Model file for the job. Use its own axes, mm. A direction names the side the tool comes from. Round coordinates to 2 decimals unless told otherwise and drop trailing zeros. Loops run counter-clockwise (first coordinate to the right, second up) from the corner with the lowest first, then second, coordinate; pieces in that order, holes last. Notation, with made-up numbers: M 27,61.5 L 35,61.5 A13 cw 35,78.5 Z; hole C 77.25,77 d3. An arc over 180 degrees is marked long. Use a Markdown table: item, result. Add a question column.
Item 1: Saw through at B-B on z = -2. Write the cut outline in (x, y) (3 decimals), then the cut area to 3 significant figures.
Item 2: Tool access for faces 1 (the flat face through (25, 2, -23)), 2 (the cylindrical face through (1.19, 5.42, -24.05)), 3 (the flat face through (48, 7, -12)): list every direction of +Z, -Z, +X, -X, +Y, -Y with a clear straight run to the whole face (end or side of a thin tool).
Item 3: Saw through at A-A on y = 2.5. Write the cut outline in (x, z) (3 decimals).
Item 4: Saw through at D-D on y = 5.5. Write the cut outline in (x, z) (3 decimals), then the cut area to 3 significant figures.
Item 5: Pin check, flat tips, straight feed: P1, Ø4, axis at x = 48, z = -2, coming from the +Y side; P2, Ø2, axis at x = 26.5, z = -20.5, coming from the -Y side; P3, Ø4, axis at y = 1.5, z = -18, coming from the -X side; P4, Ø1.6, axis at x = 49, y = 12, coming from the +Z side. Stop position of each tip, or through.
Item 6: Wall check: L1, parallel to X at y = 4.75, z = -23 (3 decimals); L2, parallel to Z at x = 37, y = 4; L3, parallel to X at y = 8, z = -22.25. Give the ranges that are in metal, low to high. Write a range as from..to.
Item 7: Saw through at C-C on x = 5. Write the cut outline in (y, z), then the cut area to 3 significant figures.
Item 8: Two-plate mould, pull along Z, no slides. Class faces 4 (the flat face through (25, 0, -7)), 5 (the flat face through (49, 13, -18.5)), 6 (the flat face through (25, 5, 0)), 7 (the cylindrical face through (24.678, 8.879, -15.996)): +Z half, -Z half, draft (parallel to the pull), parting line (faces both ways), or undercut.
```python
from build123d import *

# Parameters (mm, degrees)
SKETCH1_W           = 50
SKETCH1_H           = 25
SKETCH1_R           = 1.325
SKETCH1_W_2         = 46
SKETCH1_H_2         = 10
BOSS_EXTRUDE1_DEPTH = 7
SKETCH2_W           = 50
SKETCH2_H           = 25
SKETCH2_R           = 1.325
SKETCH2_W_2         = 46
SKETCH2_H_2         = 4
BOSS_EXTRUDE2_DEPTH = 4
SKETCH3_W           = 2
SKETCH3_H           = 12
BOSS_EXTRUDE3_DEPTH = 4
FILLET1_R           = 10
FILLET2_R           = 10
CUT_EXTRUDE1_DEPTH  = 4


with BuildPart() as part:
    # Sketch1 → Boss-Extrude1 (new body)
    with BuildSketch(Plane(origin=(0, 0, 0), x_dir=(1, 0, 0), z_dir=(0, 1, 0))):
        with Locations((25, 12.5)):
            Rectangle(SKETCH1_W, SKETCH1_H)
        with Locations(Location((2, 23, 0), (0, 0, 270))):
            Circle(SKETCH1_R, mode=Mode.SUBTRACT)
        with Locations(Location((48, 23, 0), (0, 0, 270))):
            Circle(SKETCH1_R, mode=Mode.SUBTRACT)
        with Locations(Location((48, 2, 0), (0, 0, 270))):
            Circle(SKETCH1_R, mode=Mode.SUBTRACT)
        with Locations(Location((2, 2, 0), (0, 0, 270))):
            Circle(SKETCH1_R, mode=Mode.SUBTRACT)
        with Locations((25, 12.5)):
            Rectangle(SKETCH1_W_2, SKETCH1_H_2, mode=Mode.SUBTRACT)
    extrude(amount=BOSS_EXTRUDE1_DEPTH)

    # Sketch2 → Boss-Extrude2 (add)
    with BuildSketch(Plane(origin=(0, 7, 0), x_dir=(1, 0, 0), z_dir=(0, 1, 0))):
        with Locations((25, 12.5)):
            Rectangle(SKETCH2_W, SKETCH2_H)
        with Locations(Location((2, 23, 0), (0, 0, 270))):
            Circle(SKETCH2_R, mode=Mode.SUBTRACT)
        with Locations(Location((48, 23, 0), (0, 0, 270))):
            Circle(SKETCH2_R, mode=Mode.SUBTRACT)
        with Locations(Location((48, 2, 0), (0, 0, 270))):
            Circle(SKETCH2_R, mode=Mode.SUBTRACT)
        with Locations(Location((2, 2, 0), (0, 0, 270))):
            Circle(SKETCH2_R, mode=Mode.SUBTRACT)
        with Locations((25, 12.5)):
            Rectangle(SKETCH2_W_2, SKETCH2_H_2, mode=Mode.SUBTRACT)
    extrude(amount=BOSS_EXTRUDE2_DEPTH)

    # Sketch3 → Boss-Extrude3 (add)
    with BuildSketch(Plane(origin=(0, 11, 0), x_dir=(1, 0, 0), z_dir=(0, 1, 0))):
        with Locations((49, 12.5)):
            Rectangle(SKETCH3_W, SKETCH3_H)
    extrude(amount=BOSS_EXTRUDE3_DEPTH)

    # Fillet1
    # the kernel refuses this fillet: 10 mm, written as the material it takes off along each edge
    with BuildSketch(Plane(origin=(2, 7, -14.5), x_dir=(0, 1, 0), z_dir=(1, 0, 0))) as fillet1_piece_1:
        with BuildLine():
            CenterArc((7.141428429, -10), FILLET1_R, 90, 45.572995999)
            Line((0, -3), (0, 0))
            Line((0, 0), (7.141428429, 0))
        make_face()
    extrude(amount=46, mode=Mode.SUBTRACT)

    # Fillet2
    # the kernel refuses this fillet: 10 mm, written as the material it takes off along each edge
    with BuildSketch(Plane(origin=(48, 7, -10.5), x_dir=(0, 1, 0), z_dir=(-1, 0, 0))) as fillet2_piece_1:
        with BuildLine():
            CenterArc((7.141428429, -10), FILLET2_R, 90, 45.572995999)
            Line((0, -3), (0, 0))
            Line((0, 0), (7.141428429, 0))
        make_face()
    extrude(amount=46, mode=Mode.SUBTRACT)

    # Sketch6 → Cut-Extrude1 (cut)
    with BuildSketch(Plane(origin=(0, 0, 0), x_dir=(-1, 0, 0), z_dir=(0, -1, 0))):
        with BuildLine():
            Line((-20.5, 19), (-29.5, 19))
            ThreePointArc((-29.5, 19), (-31.5, 21), (-29.5, 23))
            Line((-29.5, 23), (-20.5, 23))
            ThreePointArc((-20.5, 23), (-18.5, 21), (-20.5, 19))
        make_face()
    extrude(amount=-CUT_EXTRUDE1_DEPTH, mode=Mode.SUBTRACT)


solid = part.part
```
Entries:
| question | item | result |
|---|---|---|
| 1 | outline | M 0,0 L 0.675,0 L 0.675,11 L 0,11 Z; M 3.325,0 L 46.675,0 L 46.675,11 L 3.325,11 Z; M 49.325,0 L 50,0 L 50,11 L 49.325,11 Z |
| 1 | area | 492 mm2 |
| 2 | face 1 | -Y |
| 2 | face 2 | +Y, -Y |
| 2 | face 3 | none |
| 3 | outline | M 0,-25 L 50,-25 L 50,0 L 0,0 Z; hole C 2,-23 d2.65; hole C 2,-2 d2.65; hole M 2,-17.5 L 48,-17.5 L 48,-7.5 L 2,-7.5 Z; hole M 20.5,-23 L 29.5,-23 A2 ccw 29.5,-19 L 20.5,-19 A2 ccw Z; hole C 48,-23 d2.65; hole C 48,-2 d2.65 |
| 4 | outline | M 0,-25 L 50,-25 L 50,0 L 0,0 Z; hole C 2,-23 d2.65; hole C 2,-2 d2.65; hole M 2,-17.5 L 48,-17.5 L 48,-7.5 L 2,-7.5 Z; hole C 48,-23 d2.65; hole C 48,-2 d2.65 |
| 4 | area | 768 mm2 |
| 5 | P1 | y = 11 |
| 5 | P2 | y = 4 |
| 5 | P3 | x = 0 |
| 5 | P4 | z = -6.5 |
| 6 | L1 | 0..0.675, 3.325..46.675, 49.325..50 |
| 6 | L2 | -25..-17.5, -7.5..0 |
| 6 | L3 | 0..0.91, 3.09..46.91, 49.09..50 |
| 7 | outline | M 0,-25 L 11,-25 L 11,-15.01 A10 ccw 7,-17.5 L 0,-17.5 Z; M 0,-7.5 L 7,-7.5 A10 ccw 11,-9.99 L 11,0 L 0,0 Z |
| 7 | area | 177 mm2 |
| 8 | face 4 | draft |
| 8 | face 5 | -Z half |
| 8 | face 6 | +Z half |
| 8 | face 7 | undercut |
